Read the model definition and answer for the solid it produces. Units are mm, in the model's axes. A direction names the side the tool comes from. Give positions to 0.01 mm unless a question says otherwise; leave off trailing zeros. Write each loop counter-clockwise with the first axis right and the second up, starting at its lowest first coordinate (ties: lowest second). Pieces come first, ordered by that corner, then holes. Notation, with made-up numbers: (-21.5, 24.25) -> (-17.5, 24.25) arc R18 cw to (-17.5, 33.25) -> close; hole circle Ø7 at (23, 24.5). An arc over 180 degrees is marked (long way). Write item = value, one per line.
from build123d import *

# Parameters (mm, degrees)
SKETCH1_W                  = 55
SKETCH1_H                  = 10.2
BOSS_EXTRUDE1_DEPTH        = 6.25
F_4_0_4_DIAMETER_HOLE1_D   = 4
F_2_5_2_5_DIAMETER_HOLE1_D = 2.5
SKETCH6_W                  = 2
SKETCH6_H                  = 0.7
CUT_EXTRUDE1_DEPTH         = 56


with BuildPart() as part:
    # Sketch1 → Boss-Extrude1 (new body)
    with BuildSketch(Plane(origin=(0, 0, 0), x_dir=(1, 0, 0), z_dir=(0, 1, 0))):
        with Locations((27.5, 5.1)):
            Rectangle(SKETCH1_W, SKETCH1_H)
    extrude(amount=BOSS_EXTRUDE1_DEPTH)

    # Ø4.0 (4) Diameter Hole1 (through all)
    with Locations(Plane.XY):
        with Locations((7, 3.125), (48, 3.125)):
            Hole(F_4_0_4_DIAMETER_HOLE1_D / 2)

    # Ø2.5 (2.5) Diameter Hole1 (through all)
    with Locations(Plane(origin=(0, 6.25, 0), x_dir=(-1, 0, 0), z_dir=(0, 1, 0))):
        with Locations((-12.5, -5.1), (-42.5, -5.1)):
            Hole(F_2_5_2_5_DIAMETER_HOLE1_D / 2)

    # Sketch6 → Cut-Extrude1 (cut, through all)
    with BuildSketch(Plane(origin=(55, 0, 0), x_dir=(0, 0, -1), z_dir=(1, 0, 0))):
        with Locations((9.2, 0.35)):
            Rectangle(SKETCH6_W, SKETCH6_H)
    extrude(amount=-CUT_EXTRUDE1_DEPTH, mode=Mode.SUBTRACT)


solid = part.part
(1) The part is cut by section B-B on z = -5.1. Determine the outline of the cut face in (x, y) (3 decimals).
Checks:
outline = (0, 0) -> (11.25, 0) -> (11.25, 6.25) -> (0, 6.25) -> close; (13.75, 0) -> (41.25, 0) -> (41.25, 6.25) -> (13.75, 6.25) -> close; (43.75, 0) -> (55, 0) -> (55, 6.25) -> (43.75, 6.25) -> close; hole circle Ø4 at (7, 3.125); hole circle Ø4 at (48, 3.125)
(2) Given P1, Ø2, axis at x = 42.5, z = -5.1, coming from the +Y side; P2, Ø0.6, axis at x = 20, z = -9, coming from the -Y side, each flat-ended and moving along its own axis, determine where each tip first touches the part or whether it passes through.
Checks:
P1 = through
P2 = 0.7
(3) For a pull along X with two mould halves and no side action, classify faces 1 (the cylindrical face through (41.25, 3.08, -5.05)), 2 (the flat face through (27, 3, -10.2)), 3 (the flat face through (55, 3, -5)) as released by +X, released by -X, zero draft, split by the parting line, or undercut.
Checks:
face_1 = undercut
face_2 = zero draft
face_3 = released by +X
(4) The part is cut by section A-A on x = 48. Determine the outline of the cut face in (y, z) (3 decimals), plus the area to 4 significant figures.
Checks:
outline = (0, -8.2) -> (0.7, -8.2) -> (0.7, -10.2) -> (1.125, -10.2) -> (1.125, 0) -> (0, 0) -> close; (5.125, -10.2) -> (6.25, -10.2) -> (6.25, 0) -> (5.125, 0) -> close
area = 21.55 mm²
(5) The part is cut by section C-C on x = 12.5. Determine the outline of the cut face in (y, z), plus the area to 3 significant figures.
Checks:
outline = (0, -8.2) -> (0.7, -8.2) -> (0.7, -10.2) -> (6.25, -10.2) -> (6.25, -6.35) -> (0, -6.35) -> close; (0, -3.85) -> (6.25, -3.85) -> (6.25, 0) -> (0, 0) -> close
area = 46.7 mm²
(6) A tool of negligible diameter and unlimited length cuts with its end or side. For faces 4 (the flat face through (27, 0, -4)), 5 (the flat face through (28, 0.7, -9)), from which of +Z, -Z, +X, -X, +Y, -Y can it reach the whole face along a straight path? Write none if from no direction.
Checks:
face_4 = +Z, -Z, +X, -X, -Y
face_5 = -Z, +X, -X, -Y
(7) The part is cut by section D-D on x = 38.5. Determine the outline of the cut face in (y, z).
Checks:
outline = (0, -8.2) -> (0.7, -8.2) -> (0.7, -10.2) -> (6.25, -10.2) -> (6.25, 0) -> (0, 0) -> close
(8) Consider L1, parallel to X at y = 3, z = -1; L2, parallel to Y at x = 48, z = -7.5 (3 decimals); L3, parallel to X at y = 4.5, z = -4.5. Determine where each line is inside the solid, lowest interval first.
Checks:
L1 = 0 to 5, 9 to 46, 50 to 55
L2 = 0 to 1.125, 5.125 to 6.25
L3 = 0 to 5.55, 8.45 to 11.4, 13.6 to 41.4, 43.6 to 46.55, 49.45 to 55
